Work out the finished part from the listing and answer in its coordinate system (mm). A direction names the side the tool comes from. Round coordinates to 2 decimals unless told otherwise and drop trailing zeros. Loops run counter-clockwise (first coordinate to the right, second up) from the corner with the lowest first, then second, coordinate; pieces in that order, holes last.
from build123d import *

# Parameters (mm, degrees)
CROQUIS1_W                   = 65
CROQUIS1_H                   = 30
SALIENTE_EXTRUIR1_DEPTH      = 5
SALIENTE_EXTRUIR2_DEPTH      = 10
REDONDEO1_R                  = 5
CROQUIS3_R                   = 1.5
CORTAR_EXTRUIR1_DEPTH        = 38
CROQUIS4_R                   = 1.5
CORTAR_EXTRUIR2_DEPTH        = 31
TALADROAVANZADO1_OUTLINE_R   = 1.7
TALADROAVANZADO1_DEPTH       = 1.66
TALADROAVANZADO1_DRAFT       = -45
TALADROAVANZADO1_2_OUTLINE_R = 1.7
TALADROAVANZADO1_2_DEPTH     = 1.66
TALADROAVANZADO1_2_DRAFT     = -45
SALIENTE_EXTRUIR3_DEPTH      = 5
REDONDEO2_START              = 19.038575289
REDONDEO2_DEPTH              = 30.635489066
REDONDEO2_2_ANGLE            = 136.254425


with BuildPart() as part:
    # Croquis1 → Saliente-Extruir1 (new body)
    with BuildSketch(Plane(origin=(0, 0, 0), x_dir=(1, 0, 0), z_dir=(0, 1, 0))):
        with Locations((32.5, 15)):
            Rectangle(CROQUIS1_W, CROQUIS1_H)
    extrude(amount=SALIENTE_EXTRUIR1_DEPTH)

    # Croquis2 → Saliente-Extruir2 (add)
    with BuildSketch(Plane(origin=(0, 5, 0), x_dir=(1, 0, 0), z_dir=(0, 1, 0))):
        Polygon((2, 2), (2, 28), (65, 28), (65, 30), (0, 30), (0, 0), (65, 0), (65, 2), align=None)
    extrude(amount=SALIENTE_EXTRUIR2_DEPTH)

    # Redondeo1
    # the kernel refuses this fillet: 5 mm, written as the material it takes off along each edge
    with BuildSketch(Plane(origin=(65, 15, 12.5), x_dir=(0, -1, 0), z_dir=(0, 0, -1)), Plane(origin=(65, 15, -15.5), x_dir=(0, -1, 0), z_dir=(0, 0, -1))) as redondeo1_piece_1:
        with BuildLine():
            CenterArc((REDONDEO1_R, REDONDEO1_R), REDONDEO1_R, 180, 90)
            Line((0, REDONDEO1_R), (0, 0))
            Line((0, 0), (REDONDEO1_R, 0))
        make_face()
    extrude(amount=27, mode=Mode.SUBTRACT)
    with BuildSketch(Plane(origin=(0, 15, -42.5), x_dir=(1, 0, 0), z_dir=(0, 0, 1))) as redondeo1_piece_2:
        with BuildLine():
            CenterArc((REDONDEO1_R, -REDONDEO1_R), REDONDEO1_R, 90, 90)
            Line((0, -REDONDEO1_R), (0, 0))
            Line((0, 0), (REDONDEO1_R, 0))
        make_face()
    extrude(amount=55, mode=Mode.SUBTRACT)

    # Croquis3 → Cortar-Extruir1 (cut)
    with BuildSketch(Plane.XY):
        with Locations(Location((61, 11, 0), (0, 0, 180))):
            Circle(CROQUIS3_R)
    extrude(amount=-CORTAR_EXTRUIR1_DEPTH, mode=Mode.SUBTRACT)

    # Croquis4 → Cortar-Extruir2 (cut)
    with BuildSketch(Plane(origin=(0, 5, 0), x_dir=(1, 0, 0), z_dir=(0, 1, 0))):
        with Locations(Location((57.5, 15, 0), (0, 0, 270))):
            Circle(CROQUIS4_R)
        with Locations(Location((10, 15, 0), (0, 0, 270))):
            Circle(CROQUIS4_R)
    extrude(amount=-CORTAR_EXTRUIR2_DEPTH, mode=Mode.SUBTRACT)


with BuildPart() as taladroavanzado1_tool:
    # TaladroAvanzado1: read off the stored shape, not the designer's step
    # TaladroAvanzado1 outline → TaladroAvanzado1 (with draft: the straight prism first)
    with BuildSketch(Plane(origin=(0, 3.34, 0), x_dir=(1, 0, 0), z_dir=(0, 1, 0))):
        with Locations((57.5, 15)):
            Circle(TALADROAVANZADO1_OUTLINE_R)
        with BuildLine():
            ThreePointArc((57.5, 16.5), (59, 15), (57.5, 13.5))
            ThreePointArc((57.5, 13.5), (56, 15), (57.5, 16.5))
        make_face(mode=Mode.SUBTRACT)
    extrude(amount=TALADROAVANZADO1_DEPTH)
    # TaladroAvanzado1: the draft: its side faces are tilted about the plane it starts from
    taladroavanzado1_sides = [taladroavanzado1_tool.faces().sort_by_distance(p)[0] for p in [
        (55.8, 4.17, -15),
        (57.5, 4.17, -13.5),
    ]]
    draft(taladroavanzado1_sides, Plane(origin=(0, 3.34, 0), x_dir=(1, 0, 0), z_dir=(0, 1, 0)), TALADROAVANZADO1_DRAFT)


with BuildPart() as part_1:
    add(part.part)

    # TaladroAvanzado1: cut by taladroavanzado1_tool
    add(taladroavanzado1_tool.part, mode=Mode.SUBTRACT)


with BuildPart() as taladroavanzado1_2_tool:
    # TaladroAvanzado1 2 outline → TaladroAvanzado1 2 (with draft: the straight prism first)
    with BuildSketch(Plane(origin=(0, 3.34, 0), x_dir=(1, 0, 0), z_dir=(0, 1, 0))):
        with Locations((10, 15)):
            Circle(TALADROAVANZADO1_2_OUTLINE_R)
        with BuildLine():
            ThreePointArc((10, 16.5), (11.5, 15), (10, 13.5))
            ThreePointArc((10, 13.5), (8.5, 15), (10, 16.5))
        make_face(mode=Mode.SUBTRACT)
    extrude(amount=TALADROAVANZADO1_2_DEPTH)
    # TaladroAvanzado1 2: the draft: its side faces are tilted about the plane it starts from
    taladroavanzado1_2_sides = [taladroavanzado1_2_tool.faces().sort_by_distance(p)[0] for p in [
        (8.3, 4.17, -15),
        (10, 4.17, -13.5),
    ]]
    draft(taladroavanzado1_2_sides, Plane(origin=(0, 3.34, 0), x_dir=(1, 0, 0), z_dir=(0, 1, 0)), TALADROAVANZADO1_2_DRAFT)


with BuildPart() as part_2:
    add(part_1.part)

    # TaladroAvanzado1 2: cut by taladroavanzado1_2_tool
    add(taladroavanzado1_2_tool.part, mode=Mode.SUBTRACT)

    # Croquis7 → Saliente-Extruir3 (add)
    with BuildSketch(Plane.XY):
        with BuildLine():
            Line((47.279462763, 6.385199117), (54.355438457, 15))
            Line((54.355438457, 15), (20, 15))
            ThreePointArc((20, 15), (29.411793924, 1.079800546), (45.83626038, 4.62814091))
            Line((45.83626038, 4.62814091), (47.279462763, 6.385199117))
        make_face()
    extrude(amount=SALIENTE_EXTRUIR3_DEPTH)

    # Redondeo2: read off the stored shape, not the designer's step
    # Redondeo2 outline → Redondeo2 (cut)
    with BuildSketch(Plane(origin=(0, 0, 0), x_dir=(0.7727468393506849, -0.6347143627440037, 0), z_dir=(0.6347143627440038, 0.7727468393506848, 0)).offset(REDONDEO2_START)):
        with BuildLine():
            Line((32.482277828, -5), (32.482277828, -2))
            ThreePointArc((32.482277828, -2), (31.603598172, -4.121320344), (29.482277828, -5))
            Line((29.482277828, -5), (32.482277828, -5))
        make_face()
    extrude(amount=REDONDEO2_DEPTH, mode=Mode.SUBTRACT)

    # Redondeo2 2 outline → Redondeo2 2 (revolve, cut)
    with BuildSketch(Plane(origin=(35, 15, 0), x_dir=(-1, 0, 0), z_dir=(0, 1, 0))):
        with BuildLine():
            ThreePointArc((12, 5), (14.121320344, 4.121320344), (15, 2))
            Line((15, 2), (15, 5))
            Line((15, 5), (12, 5))
        make_face()
    revolve(axis=Axis((35, 15, 0), (0, 0, 1)), revolution_arc=REDONDEO2_2_ANGLE, mode=Mode.SUBTRACT)


solid = part_2.part
Item 1: Section B-B, the plane x = 57.5 is taken. Give the vertices of the cut face in (y, z).
Item 2: Section A-A, the plane z = -15 is taken. Give the vertices of the cut face in (x, y).
Item 3: Determine the mould class of faces 1 (the face through (33, 15, 1)), 2 (the face through (2, 9, -15)), 3 (the face through (56, 6, 0)), 4 (the face through (10.07, 1.69, -16.5)) for opening direction Z: pulls with the +Z half, pulls with the -Z half, needs draft (parallel to the pull), parting line crosses it, or undercut.
Item 4: Section D-D, the plane y = 2.25 is taken. State how many separate pieces and enclosed holes the cut face has, plus the area to 3 significant figures.
Item 5: Section C-C, the plane x = 16 is taken. Give the vertices of the cut face in (y, z), plus the area to 3 significant figures.
Item 6: Straight lines are drawn through the part: line 1 (X direction, y = 2.2, z = -15); line 2 (Z direction, x = 4.5, y = 9.75); line 3 (Z direction, x = 57.5, y = 1.75). For each, find the intervals that lie inside material, in ascending order.
Item 7: Each of these flat-tipped pins is pushed along its axis until it touches: P1, Ø4.5, axis at x = 51, y = 6.5, coming from the +Z side; P2, Ø12, axis at x = 15, z = -9, coming from the +Y side; P3, Ø3.5, axis at x = 58.5, z = -15.5, coming from the +Y side. Where does it stop, or does it pass through?
Item 8: For faces 5 (the face through (29.181, 1.175, 0.986)), 6 (the face through (33, 5, -15)), 7 (the face through (13, 7, 0)), 8 (the face through (59.614, 11.575, -28.986)), 9 (the face through (63, 14, -29)), determine the directions among +Z, -Z, +X, -X, +Y, -Y from which every point of the face is accessible in a straight line to the end or side of a thin tool.
Answer below:
1. outline: (0, -30) - (15, -30) - (15, -28) - (5, -28) - (5, -18.36) - (3.34, -16.7) - (3.34, -16.5) - (0, -16.5) - close; (0, -13.5) - (3.34, -13.5) - (3.34, -13.3) - (5, -11.64) - (5, -2) - (15, -2) - (15, 0) - (0, 0) - close
2. outline: (0, 0) - (8.5, 0) - (8.5, 3.34) - (8.3, 3.34) - (6.64, 5) - (2, 5) - (2, 14) arc R5 ccw to (0, 10) - close; (11.5, 0) - (56, 0) - (56, 3.34) - (55.8, 3.34) - (54.14, 5) - (13.36, 5) - (11.7, 3.34) - (11.5, 3.34) - close; (59, 0) - (65, 0) - (65, 5) - (60.86, 5) - (59.2, 3.34) - (59, 3.34) - close
3. face 1: needs draft
3. face 2: undercut
3. face 3: pulls with the +Z half
3. face 4: undercut
4. separate pieces: 1
4. enclosed holes: 2
4. area: 2,010 mm2
5. outline: (0, -30) - (15, -30) - (15, -28) - (5, -28) - (5, -2) - (15, -2) - (15, 0) - (0, 0) - close
5. area: 190 mm2
6. line 1: x = 0 to 8.5, 11.5 to 56, 59 to 65
6. line 2: z = -30 to -28, -2 to 0
6. line 3: z = -30 to -16.5, -13.5 to 0
7. P1: stops at z = 0
7. P2: stops at y = 5
7. P3: stops at y = 4.51
8. face 5: +Z, -Y
8. face 6: +X, +Y
8. face 7: +Z, -X, -Y
8. face 8: +Z, -Z
8. face 9: +Z, -Z, +X, +Y
